Read the model definition and answer for the solid it produces. Units are mm, in the model's axes. Face numbers are marked on the shaded views. A direction names the side the tool comes from. Coordinates: 2 decimals unless noted, no trailing zeros. Write each loop counter-clockwise with the first axis right and the second up, starting at its lowest first coordinate (ties: lowest second). Pieces come first, ordered by that corner, then holes. Notation, with made-up numbers: (54.25, -29) -> (73.25, -29) arc R22 cw to (73.25, 10) -> close; hole circle Ø7 at (87, -20.5). An arc over 180 degrees is marked (long way). Use CSV: the item, a comma, the result in double quotes. Start each with the question number.
from build123d import *

# Parameters (mm, degrees)
F0_W        = 22.098
F0_H        = 43.688
F1_DEPTH    = 25.4
F2_T1_DEPTH = 50.8
F3_R        = 5.588


# Not quite as in the source:
# - a fillet or chamfer that OpenCascade refuses, or shapes differently, is made with other operations: its cross-section is extruded or revolved along the edge and cut away or added


with BuildPart() as f1:
    # F0 (on Top) → F1 (new body)
    with BuildSketch(Plane.XY):
        Polygon((21.844, -26.924), (21.844, 26.924), (-21.844, 26.924), (-21.844, 0), (-16.764, 0), (-16.764, 21.844), (-10.414, 21.844), (-10.414, -26.924), align=None)
        with Locations((5.715, 0)):
            Rectangle(F0_W, F0_H, mode=Mode.SUBTRACT)
    extrude(amount=F1_DEPTH)

    # F2: fillet of radius 5.08 on 6 edges, made by hand

    # F2_s2 → F2_t1 (cut)
    with BuildSketch(Plane.XY.offset(-12.7)):
        with BuildLine():
            ThreePointArc((-16.764, 26.924), (-20.3561024484, 25.4361024484), (-21.844, 21.844))
            Line((-21.844, 21.844), (-21.844, 26.924))
            Line((-21.844, 26.924), (-16.764, 26.924))
        make_face()
        with BuildLine():
            ThreePointArc((21.844, 21.844), (20.3561024484, 25.4361024484), (16.764, 26.924))
            Line((16.764, 26.924), (21.844, 26.924))
            Line((21.844, 26.924), (21.844, 21.844))
        make_face()
        with BuildLine():
            ThreePointArc((-5.334, -26.924), (-8.9261024484, -25.4361024484), (-10.414, -21.844))
            Line((-10.414, -21.844), (-10.414, -26.924))
            Line((-10.414, -26.924), (-5.334, -26.924))
        make_face()
        with BuildLine():
            ThreePointArc((16.764, -26.924), (20.3561024484, -25.4361024484), (21.844, -21.844))
            Line((21.844, -21.844), (21.844, -26.924))
            Line((21.844, -26.924), (16.764, -26.924))
        make_face()
        with BuildLine():
            ThreePointArc((-21.844, 0), (-18.2518975516, 1.4878975516), (-16.764, 5.08))
            Line((-16.764, 5.08), (-16.764, 0))
            Line((-16.764, 0), (-21.844, 0))
        make_face()
        with BuildLine():
            ThreePointArc((-21.844, 5.08), (-20.3561024484, 1.4878975516), (-16.764, 0))
            Line((-16.764, 0), (-21.844, 0))
            Line((-21.844, 0), (-21.844, 5.08))
        make_face()
    extrude(amount=F2_T1_DEPTH, mode=Mode.SUBTRACT)

    # F3
    f3_edges = [f1.edges().sort_by_distance(p)[0] for p in [
        (-5.334, -21.844, 12.7),
        (16.764, -21.844, 12.7),
        (16.764, 21.844, 12.7),
        (-5.334, 21.844, 12.7),
    ]]
    fillet(f3_edges, radius=F3_R)


solid = f1.part
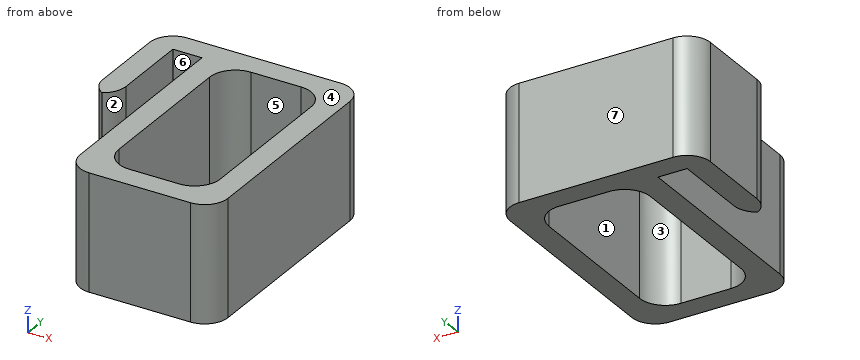
1) Find the intervals of material crossed by line 1 along X through (y, z) = (11, 12.25); line 2 along X through (y, z) = (-8.5, 24); line 3 along Y through (x, z) = (9.5, 17), in increasing order.
2) Which of the six approach directions +Z, -Z, +X, -X, +Y, -Y give full straight-line access (tool end or side, diameter ignored) to the marked faces 5, 6 and 7?
3) The mould has two halves that part along Y. Classify the marked faces 1, 2, 3 and 4: pulls with the +Y half, pulls with the -Y half, needs draft (parallel to the pull), parting line crosses it, or undercut.
4) This flat-tipped pin is pushed along its axis until it touches: pin 1 (3 mm diameter, centred on x = -14, z = 18.5, fed in from -Y). Where does it stop, or does it pass through?
5) Section C-C, the plane z = 7.5 is taken. Give the vertices of the cut face in (x, y).
6) Section D-D, the plane y = 14.5 is taken. Give the vertices of the cut face in (x, z).
7) Section A-A, the plane y = -10.5 is taken. Give the vertices of the cut face in (x, z), plus the area to 3 significant figures.
8) Section B-B, the plane x = 9 is taken. Give the vertices of the cut face in (y, z), plus the area to 3 significant figures.
The answers:
1,line 1,"x = -21.84 to -16.76, -10.41 to -5.33, 16.76 to 21.84"
1,line 2,"x = -10.41 to -5.33, 16.76 to 21.84"
1,line 3,"y = -26.92 to -21.84, 21.84 to 26.92"
2,face 5,"+Z, -Z"
2,face 6,"+Z, -Z, -Y"
2,face 7,"+Z, -Z, +X, -X, +Y"
3,face 1,"undercut"
3,face 2,"pulls with the -Y half"
3,face 3,"undercut"
3,face 4,"needs draft"
4,pin 1,"stops at y = 21.84"
5,outline,"(-21.84, 5.08) arc R5.08 ccw to (-19.3, 0.68) arc R5.08 ccw to (-16.76, 5.08) -> (-16.76, 21.84) -> (-10.41, 21.84) -> (-10.41, -21.84) arc R5.08 ccw to (-5.33, -26.92) -> (16.76, -26.92) arc R5.08 ccw to (21.84, -21.84) -> (21.84, 21.84) arc R5.08 ccw to (16.76, 26.92) -> (-16.76, 26.92) arc R5.08 ccw to (-21.84, 21.84) -> close; hole (-5.33, -16.26) arc R5.59 ccw to (0.25, -21.84) -> (11.18, -21.84) arc R5.59 ccw to (16.76, -16.26) -> (16.76, 16.26) arc R5.59 ccw to (11.18, 21.84) -> (0.25, 21.84) arc R5.59 ccw to (-5.33, 16.26) -> close"
6,outline,"(-21.84, 0) -> (-16.76, 0) -> (-16.76, 25.4) -> (-21.84, 25.4) -> close; (-10.41, 0) -> (-5.33, 0) -> (-5.33, 25.4) -> (-10.41, 25.4) -> close; (16.76, 0) -> (21.84, 0) -> (21.84, 25.4) -> (16.76, 25.4) -> close"
7,outline,"(-10.41, 0) -> (-5.33, 0) -> (-5.33, 25.4) -> (-10.41, 25.4) -> close; (16.76, 0) -> (21.84, 0) -> (21.84, 25.4) -> (16.76, 25.4) -> close"
7,area,"258 mm^2"
8,outline,"(-26.92, 0) -> (-21.84, 0) -> (-21.84, 25.4) -> (-26.92, 25.4) -> close; (21.84, 0) -> (26.92, 0) -> (26.92, 25.4) -> (21.84, 25.4) -> close"
8,area,"258 mm^2"
